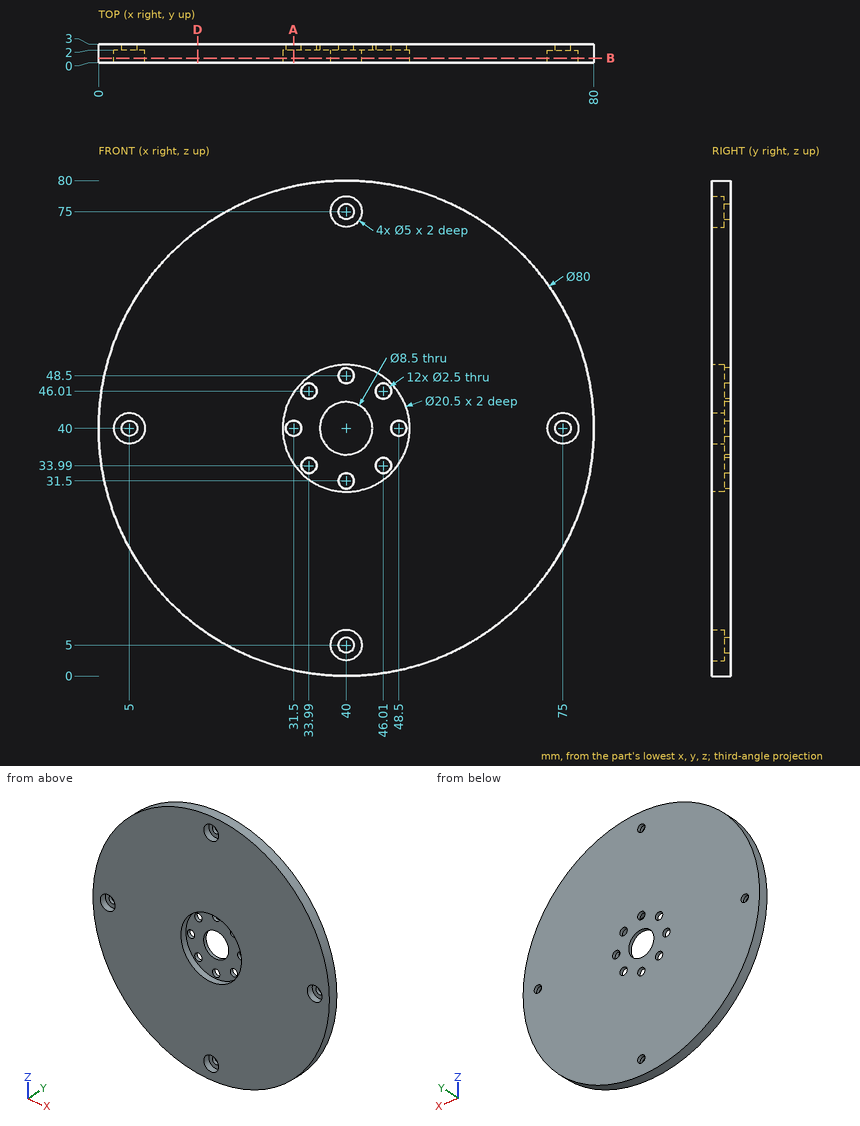
Can you work these out from the drawing? Everything is in mm from the part's minimum corner. Give positions to 0.01 mm unless a question says otherwise; leave off trailing zeros. Order: outer loops, then holes, each group sorted by start corner. A loop starts at its lowest first (then second) coordinate and runs counter-clockwise, first axis right, second up.
Item 1: If we section it at B-B, the plane y = 0.7: Write out the boundary of the cut face in (x, z), plus the area to 3 significant figures.
Item 2: If we section it at A-A, the plane x = 31.5: Write out the boundary of the cut face in (y, z), plus the area to 3 significant figures.
Item 3: I need wall thicknesses on line 1 (X direction, y = 2.1, z = 33.5); line 2 (X direction, y = 1.65, z = 40.5); line 3 (X direction, y = 1.5, z = 6.5) (1 decimal). Which ranges of each line are inside material? Lowest first, please.
Item 4: I'm going to push flat-ended pins straight in: pin 1 (4.5 mm diameter, centred on x = 40, z = 75, fed in from -Y); pin 2 (1.5 mm diameter, centred on x = 43, y = 2, fed in from +Z); pin 3 (1.5 mm diameter, centred on y = 2, z = 23.5, fed in from -X). Where does each tip first touch, or does it pass through?
Item 5: If we section it at D-D, the plane x = 16: Write out the boundary of the cut face in (y, z).
Values:
1. outline: circle Ø80 at (40, 40); hole circle Ø5 at (5, 40); hole circle Ø20.5 at (40, 40); hole circle Ø5 at (40, 5); hole circle Ø5 at (40, 75); hole circle Ø5 at (75, 40)
1. area: 4,620 mm2
2. outline: (0, 0.91) - (3, 0.91) - (3, 38.75) - (2, 38.75) - (2, 34.27) - (0, 34.27) - close; (0, 45.73) - (2, 45.73) - (2, 41.25) - (3, 41.25) - (3, 79.09) - (0, 79.09) - close
2. area: 209 mm2
3. line 1: x = 0.53 to 32.84, 35.14 to 44.86, 47.16 to 79.47
3. line 2: x = 0 to 2.55, 7.45 to 29.76, 50.24 to 72.55, 77.45 to 80
3. line 3: x = 18.1 to 38, 42 to 61.9
4. pin 1: stops at y = 2
4. pin 2: stops at z = 79.94
4. pin 3: stops at x = 3.23
5. outline: (0, 8) - (3, 8) - (3, 72) - (0, 72) - close
